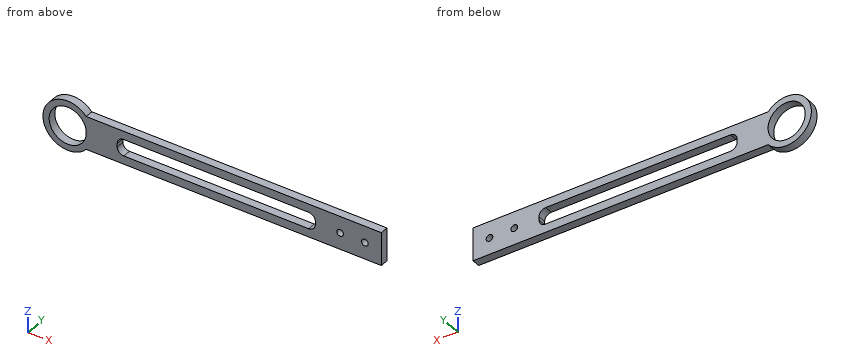
from build123d import *

# Parameters (mm, degrees)
SKETCH1_W              = 254
SKETCH1_H              = 25.4
BOSS_EXTRUDE1_DEPTH    = 3.175
FILLET1_R              = 12.7
F_10_CLEARANCE_HOLE1_D = 5.1054
SKETCH9_W              = 152.4
SKETCH9_H              = 12.7
CUT_EXTRUDE2_DEPTH     = 128.791284914
FILLET2_R              = 5.08
SKETCH11_R             = 19.05
BOSS_EXTRUDE2_DEPTH    = 6.35
SKETCH10_R             = 14.2875
CUT_EXTRUDE3_DEPTH     = 135.853429693


with BuildPart() as part:
    # Sketch1 → Boss-Extrude1 (new, symmetric)
    with BuildSketch(Plane(origin=(0, 0, 0), x_dir=(1, 0, 0), z_dir=(0, 1, 0))):
        Rectangle(SKETCH1_W, SKETCH1_H)
    extrude(amount=BOSS_EXTRUDE1_DEPTH, both=True)

    # Fillet1
    fillet1_edges = [part.edges().sort_by_distance(p)[0] for p in [
        (-127, 0, -12.7),
        (-127, 0, 12.7),
    ]]
    fillet(fillet1_edges, radius=FILLET1_R - 0.0001)  # a hair under: the kernel refuses the full size

    # #10 Clearance Hole1 (through all)
    with Locations(Plane(origin=(0, 3.175, 0), x_dir=(1, 0, 0), z_dir=(0, 1, 0))):
        with Locations((114.3, 0), (95.25, 0)):
            Hole(F_10_CLEARANCE_HOLE1_D / 2)

    # Sketch9 → Cut-Extrude2 (cut, through all)
    with BuildSketch(Plane(origin=(0, 3.175, 0), x_dir=(1, 0, 0), z_dir=(0, 1, 0))):
        Rectangle(SKETCH9_W, SKETCH9_H)
    extrude(amount=-CUT_EXTRUDE2_DEPTH, mode=Mode.SUBTRACT)

    # Fillet2
    fillet2_edges = [part.edges().sort_by_distance(p)[0] for p in [
        (76.2, 0, -6.35),
        (76.2, 0, 6.35),
        (-76.2, 0, 6.35),
        (-76.2, 0, -6.35),
    ]]
    fillet(fillet2_edges, radius=FILLET2_R)

    # Sketch11 → Boss-Extrude2 (add)
    with BuildSketch(Plane.XZ.offset(3.175)):
        with Locations((-114.3, 0)):
            Circle(SKETCH11_R)
    extrude(amount=-BOSS_EXTRUDE2_DEPTH)

    # Sketch10 → Cut-Extrude3 (cut, through all)
    with BuildSketch(Plane.XZ.offset(3.175)):
        with Locations(Location((-114.3, 0, 0), (0, 0, 270))):
            Circle(SKETCH10_R)
    extrude(amount=-CUT_EXTRUDE3_DEPTH, mode=Mode.SUBTRACT)


solid = part.part
Source: CAD feature listing. Evaluate the final solid. Frame: model axes, mm. Round coordinates to 2 decimals unless told otherwise and drop trailing zeros. Loops run counter-clockwise (first coordinate to the right, second up) from the corner with the lowest first, then second, coordinate; pieces in that order, holes last. Notation, with made-up numbers: (72.5, 29) -> (120.5, 29) arc R18 cw to (120.5, 63) -> close; hole circle Ø8 at (-8.5, 71.25). An arc over 180 degrees is marked (long way). Answer as a JSON object with one key per item and string values. Group by question number.
Q1. Ray query, line 1 (Z direction, x = 56, y = 0.25); line 2 (Z direction, x = 95.25, y = -0.5); line 3 (X direction, y = 2.75, z = 3). Return the intervals inside material, ascending. Write a range as from..to.
Q2. Section query B-B (y = 1). State how many separate pieces and enclosed holes the cut face has, plus the area to 3 significant figures.
Q3. Section query C-C (x = -64.5). Output: boundary loops of the cut face in (y, z) (3 decimals), plus the area to 3 significant figures.
Q4. Contact query for flat-ended pins moving along their axis: P1, Ø2, axis at x = 18.5, y = -1, coming from the +Z side; P2, Ø2, axis at x = -11.5, y = -1.5, coming from the -Z side; P3, Ø3, axis at x = 114.3, z = 0, coming from the -Y side; P4, Ø3, axis at y = 0, z = 0, coming from the -X side. Output: stop coordinate, or through.
Q5. Section query A-A (x = 95.25). Output: boundary loops of the cut face in (y, z) (3 decimals), plus the area to 3 significant figures.
Completed:
{
 "1": {"line 1": "-12.7..-6.35, 6.35..12.7", "line 2": "-12.7..-2.55, 2.55..12.7", "line 3": "-133.11..-128.27, -100.33..-75.9, 75.9..127"},
 "2": {"separate pieces": "1", "enclosed holes": "4", "area": "4,230 mm²"},
 "3": {"outline": "(-3.175, -12.7) -> (3.175, -12.7) -> (3.175, -6.35) -> (-3.175, -6.35) -> close; (-3.175, 6.35) -> (3.175, 6.35) -> (3.175, 12.7) -> (-3.175, 12.7) -> close", "area": "80.6 mm²"},
 "4": {"P1": "z = 12.7", "P2": "z = -12.7", "P3": "through", "P4": "x = -133.35"},
 "5": {"outline": "(-3.175, -12.7) -> (3.175, -12.7) -> (3.175, -2.553) -> (-3.175, -2.553) -> close; (-3.175, 2.553) -> (3.175, 2.553) -> (3.175, 12.7) -> (-3.175, 12.7) -> close", "area": "129 mm²"}
}
